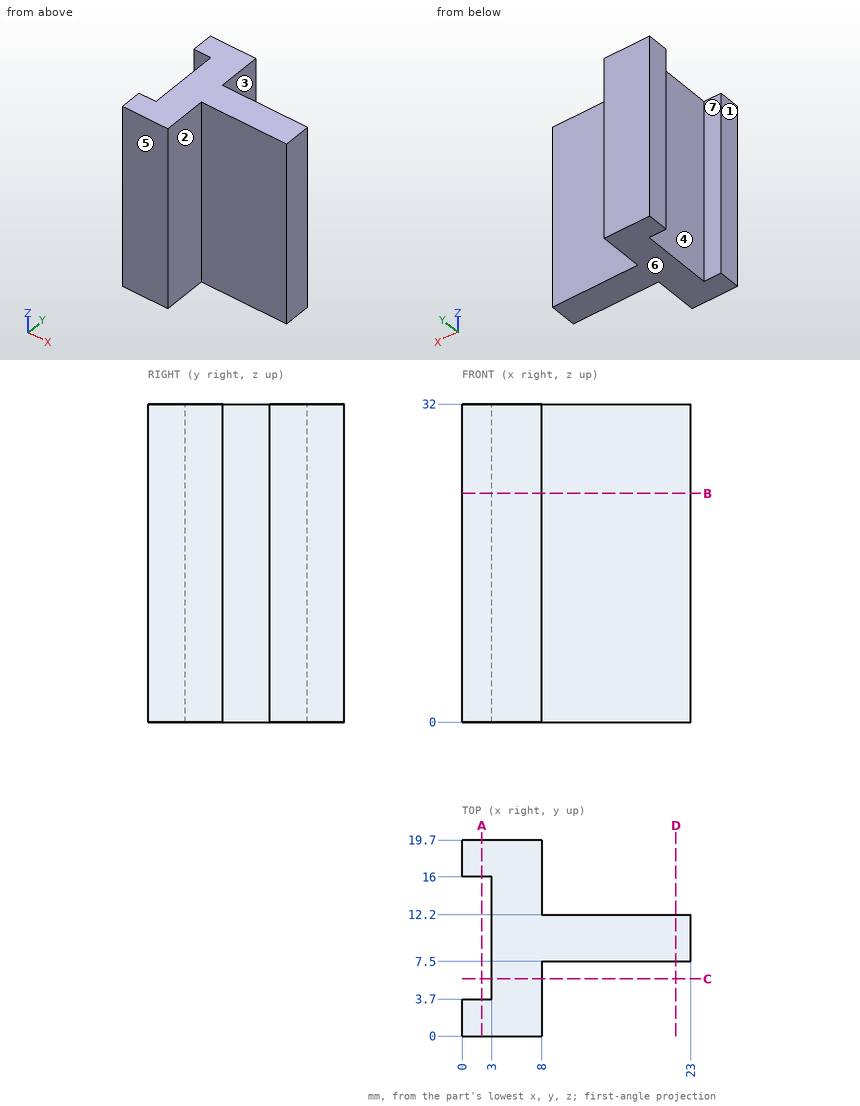
The figure shows three views and two pictorial views of one solid part (mm, origin at its lowest corner). Answer the questions. A direction names the side the tool comes from. Coordinates: 2 decimals unless noted, no trailing zeros. Loops run counter-clockwise (first coordinate to the right, second up) from the corner with the lowest first, then second, coordinate; pieces in that order, holes last. Notation, with made-up numbers: (26, 61.5) - (66, 61.5) arc R28 cw to (66, 97.5) - close; hole circle Ø1 at (76.25, -21). An arc over 180 degrees is marked (long way). Use a Markdown table: item, result. Add a question column.
1) The part is cut by section D-D, the plane x = 21.5. Give the vertices of the cut face in (y, z).
2) The part is cut by section A-A, the plane x = 2. Give the vertices of the cut face in (y, z), and give its area (3 significant figures).
3) The mould has two halves that part along Y. Classify the marked faces 5, 6 and 7: released by +Y, released by -Y, zero draft, split by the parting line, or undercut.
4) Find the intervals of material crossed by line 1 (Y direction, x = 1.5, z = 27); line 2 (Y direction, x = 13, z = 12); line 3 (X direction, y = 3.75, z = 11), in increasing order.
5) For the marked faces 1, 2, 3 and 4, determine the directions among +Z, -Z, +X, -X, +Y, -Y from which every point of the face is accessible in a straight line to the end or side of a thin tool.
6) Given pin 1 (4.5 mm diameter, centred on x = 18, z = 14, fed in from +Y); pin 2 (2 mm diameter, centred on y = 2, z = 20.5, fed in from +X); pin 3 (1 mm diameter, centred on y = 8, z = 15.5, fed in from -X), each flat-ended and moving along its own axis, determine where each tip first touches the part or whether it passes through.
7) The part is cut by section B-B, the plane z = 23. Give the vertices of the cut face in (x, y), and give its area (3 significant figures).
8) The part is cut by section C-C, the plane y = 5.75. Give the vertices of the cut face in (x, z).
Here are the results:
| question | item | result |
|---|---|---|
| 1 | outline | (7.5, 0) - (12.2, 0) - (12.2, 32) - (7.5, 32) - close |
| 2 | outline | (0, 0) - (3.7, 0) - (3.7, 32) - (0, 32) - close; (16, 0) - (19.7, 0) - (19.7, 32) - (16, 32) - close |
| 2 | area | 237 mm^2 |
| 3 | face 5 | released by -Y |
| 3 | face 6 | zero draft |
| 3 | face 7 | undercut |
| 4 | line 1 | y = 0 to 3.7, 16 to 19.7 |
| 4 | line 2 | y = 7.5 to 12.2 |
| 4 | line 3 | x = 3 to 8 |
| 5 | face 1 | +Z, -Z, -X, +Y, -Y |
| 5 | face 2 | +Z, -Z, +X, -Y |
| 5 | face 3 | +Z, -Z, +X, +Y |
| 5 | face 4 | +Z, -Z, -X |
| 6 | pin 1 | stops at y = 12.2 |
| 6 | pin 2 | stops at x = 8 |
| 6 | pin 3 | stops at x = 3 |
| 7 | outline | (0, 0) - (8, 0) - (8, 7.5) - (23, 7.5) - (23, 12.2) - (8, 12.2) - (8, 19.7) - (0, 19.7) - (0, 16) - (3, 16) - (3, 3.7) - (0, 3.7) - close |
| 7 | area | 191 mm^2 |
| 8 | outline | (3, 0) - (8, 0) - (8, 32) - (3, 32) - close |
